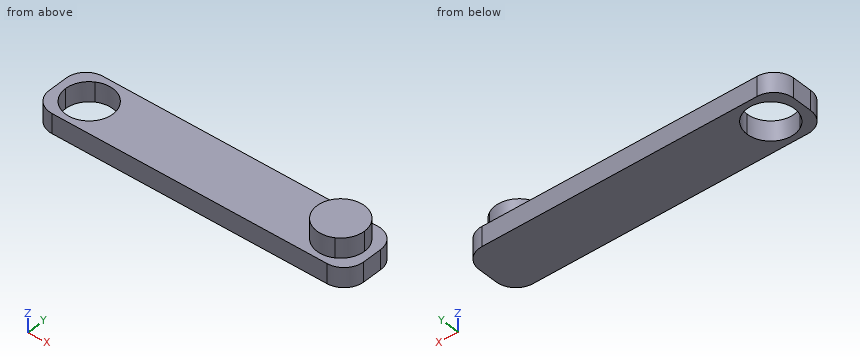
```python
from build123d import *

# Parameters (mm, degrees)
EXTRUDE_1_DEPTH = 5
EXTRUDE_2_DEPTH = 10


with BuildPart() as part:
    # Sketch 1 → Extrude 1 (new body)
    with BuildSketch(Plane.XY):
        with BuildLine():
            Line((65.989328864, 7.5), (14, 7.5))
            ThreePointArc((14, 7.5), (11, 2.303847577), (5, 2.303847577))
            Line((5, 2.303847577), (5, 0))
            Line((5, 0), (75, 0))
            Line((75, 0), (75, 2.291529254))
            ThreePointArc((75, 2.291529254), (68.991997831, 2.296146576), (65.989328864, 7.5))
        make_face()
        with BuildLine():
            ThreePointArc((5, 2.303847577), (2.803847577, 4.5), (2, 7.5))
            Line((2, 7.5), (0, 7.5))
            Line((0, 7.5), (0, 5))
            ThreePointArc((0, 5), (1.464466094, 1.464466094), (5, 0))
            Line((5, 0), (5, 2.303847577))
        make_face()
        with BuildLine():
            Line((5, 12.696152423), (5, 15))
            ThreePointArc((5, 15), (1.464466094, 13.535533906), (0, 10))
            Line((0, 10), (0, 7.5))
            Line((0, 7.5), (2, 7.5))
            ThreePointArc((2, 7.5), (2.803847577, 10.5), (5, 12.696152423))
        make_face()
        with BuildLine():
            Line((75, 15), (5, 15))
            Line((5, 15), (5, 12.696152423))
            ThreePointArc((5, 12.696152423), (11, 12.696152423), (14, 7.5))
            Line((14, 7.5), (65.989328864, 7.5))
            ThreePointArc((65.989328864, 7.5), (68.991997831, 12.703853424), (75, 12.708470746))
            Line((75, 12.708470746), (75, 15))
        make_face()
        with BuildLine():
            ThreePointArc((80, 10), (78.535533906, 13.535533906), (75, 15))
            Line((75, 15), (75, 12.708470746))
            ThreePointArc((75, 12.708470746), (77.203853424, 10.508002169), (78.010671136, 7.5))
            Line((78.010671136, 7.5), (80, 7.5))
            Line((80, 7.5), (80, 10))
        make_face()
        with BuildLine():
            Line((80, 7.5), (78.010671136, 7.5))
            ThreePointArc((78.010671136, 7.5), (77.203853424, 4.491997831), (75, 2.291529254))
            Line((75, 2.291529254), (75, 0))
            ThreePointArc((75, 0), (78.535533906, 1.464466094), (80, 5))
            Line((80, 5), (80, 7.5))
        make_face()
    extrude(amount=EXTRUDE_1_DEPTH)

    # Sketch 1_3 → Extrude 2 (add)
    with BuildSketch(Plane.XY):
        with BuildLine():
            ThreePointArc((78.010671136, 7.5), (77.203853424, 10.508002169), (75, 12.708470746))
            Line((75, 12.708470746), (75, 7.5))
            Line((75, 7.5), (78.010671136, 7.5))
        make_face()
        with BuildLine():
            Line((75, 7.5), (75, 12.708470746))
            ThreePointArc((75, 12.708470746), (68.991997831, 12.703853424), (65.989328864, 7.5))
            Line((65.989328864, 7.5), (72, 7.5))
            Line((72, 7.5), (75, 7.5))
        make_face()
        with BuildLine():
            Line((72, 7.5), (65.989328864, 7.5))
            ThreePointArc((65.989328864, 7.5), (68.991997831, 2.296146576), (75, 2.291529254))
            Line((75, 2.291529254), (75, 7.5))
            Line((75, 7.5), (72, 7.5))
        make_face()
        with BuildLine():
            Line((78.010671136, 7.5), (75, 7.5))
            Line((75, 7.5), (75, 2.291529254))
            ThreePointArc((75, 2.291529254), (77.203853424, 4.491997831), (78.010671136, 7.5))
        make_face()
    extrude(amount=EXTRUDE_2_DEPTH)


solid = part.part
```
Check sheet for the modelled part. Datum: model origin and axes. Units: mm. Coordinates: 2 decimals unless noted, no trailing zeros. Order: outer loops, then holes, each group sorted by start corner. A loop starts at its lowest first (then second) coordinate and runs counter-clockwise, first axis right, second up. Notation, with made-up numbers: (85, 22) -> (107, 22) arc R16 cw to (107, 50) -> close; hole circle Ø11 at (73, 71.5). An arc over 180 degrees is marked (long way). Write item = value, one per line. Start each with the question number.
1) Cross-section at A-A (z = 3). Enter the section's corners in (x, y), then the cut area to 3 significant figures.
2) Cross-section at D-D (x = 32). Enter the section's corners in (y, z).
3) Cross-section at C-C (y = 6). Enter the section's corners in (x, z), then the cut area to 3 significant figures.
4) Go/stop test with flat-tipped pins: P1, Ø4, axis at x = 35, y = 13, coming from the +Z side; P2, Ø1.5, axis at y = 11.5, z = 2.5, coming from the +X side. Record where each tip stops, or that it passes through.
5) Material ranges on L1, parallel to Z at x = 27.5, y = 1.25; L2, parallel to X at y = 8.75, z = 2; L3, parallel to Y at x = 10.5, z = 4, recorded low to high.
6) Cross-section at B-B (x = 11). Enter the section's corners in (y, z).
Ans:
q1.outline = (0, 5) arc R5 ccw to (5, 0) -> (75, 0) arc R5 ccw to (80, 5) -> (80, 10) arc R5 ccw to (75, 15) -> (5, 15) arc R5 ccw to (0, 10) -> close; hole circle Ø12 at (8, 7.5)
q1.area = 1,070 mm²
q2.outline = (0, 0) -> (15, 0) -> (15, 5) -> (0, 5) -> close
q3.outline = (0, 0) -> (2.19, 0) -> (2.19, 5) -> (0, 5) -> close; (13.81, 0) -> (80, 0) -> (80, 5) -> (77.82, 5) -> (77.82, 10) -> (66.18, 10) -> (66.18, 5) -> (13.81, 5) -> close
q3.area = 400 mm²
q4.P1 = 5
q4.P2 = 79.94
q5.L1 = 0 to 5
q5.L2 = 0 to 2.13, 13.87 to 80
q5.L3 = 0 to 2.05, 12.95 to 15
q6.outline = (0, 0) -> (2.3, 0) -> (2.3, 5) -> (0, 5) -> close; (12.7, 0) -> (15, 0) -> (15, 5) -> (12.7, 5) -> close
